Design review of the part built by this model. Coordinates are the model's own, in mm. A direction names the side the tool comes from. Round coordinates to 2 decimals unless told otherwise and drop trailing zeros. Loops run counter-clockwise (first coordinate to the right, second up) from the corner with the lowest first, then second, coordinate; pieces in that order, holes last. Notation, with made-up numbers: M -32,-9 L 20,-9 A23 ccw 20,19 Z; hole C -1,16.5 d9. An arc over 180 degrees is marked long. Use a Markdown table: item, result.
Autodesk Inventor part; units mm, degrees
ref_plane "YZ Plane" through (0, 0, 0) normal (1, 0, 0) x (0, 1, 0)
ref_plane "XZ Plane" through (0, 0, 0) normal (0, 1, 0) x (-1, 0, 0)
ref_plane "XY Plane" through (0, 0, 0) normal (0, 0, 1) x (1, 0, 0)
sketch "Sketch1" plane through (0, 0, 0) normal (0, 0, 1) x (1, 0, 0)
  circle A0 centre (0, 0) radius 20
  line L0 (-19.68, 3.5636) -> (-29, -47.9062)
  line L1 (19.68, 3.5636) -> (29, -47.9062)
  line L2 (9.9593, -5.75) -> (0, 0) construction
  circle A1 centre (8.4134, -4.8575) radius 2.5
  line L3 (0, 0) -> (9.9593, 5.75) construction
  line L4 (0, 0) -> (-9.9593, -5.75) construction
  circle A2 centre (-8.4134, -4.8575) radius 2.5
  circle A3 centre (0, 0) radius 9.715 construction
  circle A4 centre (0, 0) radius 11.5 construction
  circle A5 centre (0, 9.715) radius 2.5
  line L5 (0, 0) -> (-9.9593, 5.75) construction
  line L6 (11.5, 0) -> (-11.5, 0) construction
  circle A6 centre (-9.9593, 5.75) radius 4
  circle A7 centre (-9.9593, 5.75) radius 2.25
  line L7 (0, -48.5721) -> (0, 22.5) construction
  circle A8 centre (0, -11.5) radius 2.25
  circle A9 centre (0, -11.5) radius 4
  circle A10 centre (9.9593, 5.75) radius 4
  circle A11 centre (9.9593, 5.75) radius 2.25
  arc A12 (-28.2326, -43.6683) -> (28.2326, -43.6683) centre (0, 0) ccw
  arc A13 (-29, -47.9062) -> (29, -47.9062) centre (0, 0) ccw
  line L8 (8, -59.5) -> (-8, -59.5)
  line L9 (-8, -59.5) -> (-8, -52.5)
  line L10 (-8, -52.5) -> (8, -52.5)
  line L11 (8, -52.5) -> (8, -59.5)
  line L12 (8, -59.5) -> (-8, -52.5) construction
  line L13 (-8, -59.5) -> (8, -52.5) construction
  point P0 (0, 11.4686)
  point P1 (0, 11.4686)
  point P2 (11.5, 0)
  point P3 (-11.5, 0)
  point P4 (0, -56)
  dimension "d18" = 23
  dimension "d0" = 40
  dimension "d17" = 19.43
  dimension "d19" = 30
  dimension "d20" = 30
  dimension "d21" = 4.5
  dimension "d22" = 8
  dimension "d23" = 5
  dimension "d24" = 104
  dimension "d25" = 112
  dimension "d48" = 58
  dimension "d60" = 16
  dimension "d61" = 7
  dimension "d40" = 14
  dimension "d41" = 50
  dimension "d50" = 25
  dimension "d51" = 35
  dimension "d52" = 2.5
  dimension "d53" = 4
extrude "Extrusion1" add sketch "Sketch1" along normal blind 6 contours A0 | A0 L1 A12 L0 | L1 A13 L11 L10 L9 L0 A12 | A13 L9 L10 L11 | A1 | A2 | A5 | A6 | A9 | A10
extrude "Extrusion2" cut sketch "Sketch1" along normal blind 3.5 contours A6 | A9 | A10 | A11
extrude "Extrusion4" add sketch "Sketch1" along normal blind 49 from surface at 6 contours L1 A13 L11 L10 L9 L0 A12 | A13 L9 L10 L11
properties part number "thigh_hip_connector"
1. Take a section at D-D on z = 38.5. Give the boundary of the cut face in (x, y), and give its area (3 significant figures).
Check values:
| item | result |
|---|---|
| outline | M -29,-47.91 A56 ccw 29,-47.91 L 28.23,-43.67 A52 cw -28.23,-43.67 Z |
| area | 241 mm² |
2. The part is to be moulded in two halves that separate along Y. For faces 1 (the face through (0, -23, 6)), 2 (the face through (2, -13, 3.5)), 3 (the face through (0, -52, 30)), say which applies: pulls with the +Y half, pulls with the -Y half, needs draft (parallel to the pull), parting line crosses it, or undercut.
Check values:
| item | result |
|---|---|
| face 1 | needs draft |
| face 2 | undercut |
| face 3 | pulls with the +Y half |
3. Take a section at A-A on x = 0. Give the boundary of the cut face in (y, z), and give its area (3 significant figures).
Check values:
| item | result |
|---|---|
| outline | M -56,0 L -15.5,0 L -15.5,3.5 L -13.75,3.5 L -13.75,6 L -52,6 L -52,55 L -56,55 Z; M -9.25,3.5 L -7.5,3.5 L -7.5,0 L 20,0 L 20,6 L -9.25,6 Z |
| area | 613 mm² |
4. Insertion check: pin 1 (2.5 mm diameter, centred on x = -8, y = 4, fed in from -Z); pin 2 (8 mm diameter, centred on x = 9, z = 33, fed in from -Y); pin 3 (5 mm diameter, centred on x = 12.5, z = 26, fed in from +Y); pin 4 (6.5 mm diameter, centred on x = 9.5, y = 6.5, fed in from -Z). Each pin has a flat end and moves straight along its axis. Give the tip position at first contact, or say it passes through.
Check values:
| item | result |
|---|---|
| pin 1 | stops at z = 3.5 |
| pin 2 | stops at y = -55.78 |
| pin 3 | stops at y = -49.79 |
| pin 4 | stops at z = 0 |
5. Machinability: for faces 4 (the face through (11.8, 9.3, 1.7)), 5 (the face through (0, -53, 55)), which of the approach directions +Z, -Z, +X, -X, +Y, -Y give a long, thin tool a straight path to every point of the face, cutting with its end or side? Answer none if there is none.
Check values:
| item | result |
|---|---|
| face 4 | -Z |
| face 5 | +Z, +X, -X, +Y, -Y |
6. Take a section at B-B on y = -11.5. Give the boundary of the cut face in (x, z), and give its area (3 significant figures).
Check values:
| item | result |
|---|---|
| outline | M -22.41,0 L -4,0 L -4,3.5 L -2.25,3.5 L -2.25,6 L -22.41,6 Z; M 2.25,3.5 L 4,3.5 L 4,0 L 22.41,0 L 22.41,6 L 2.25,6 Z |
| area | 230 mm² |
7. Take a section at C-C on y = 5.75. Give the boundary of the cut face in (x, z), and give its area (3 significant figures).
Check values:
| item | result |
|---|---|
| outline | M -19.16,0 L -13.96,0 L -13.96,3.5 L -12.21,3.5 L -12.21,6 L -19.16,6 Z; M -7.71,3.5 L -5.96,3.5 L -5.96,0 L 5.96,0 L 5.96,3.5 L 7.71,3.5 L 7.71,6 L -7.71,6 Z; M 12.21,3.5 L 13.96,3.5 L 13.96,0 L 19.16,0 L 19.16,6 L 12.21,6 Z |
| area | 151 mm² |
8. Wall thickness on line 1 along X through (y, z) = (5, 2); line 2 along Y through (x, z) = (0, 2.35); line 3 along Z through (x, y) = (-17, -26.5): over which ranges is each line inside the solid? List them lowest first. Write a range as from..to.
Check values:
| item | result |
|---|---|
| line 1 | x = -19.36..-13.89, -6.03..6.03, 13.89..19.36 |
| line 2 | y = -56..-15.5, -7.5..20 |
| line 3 | z = 0..6 |
